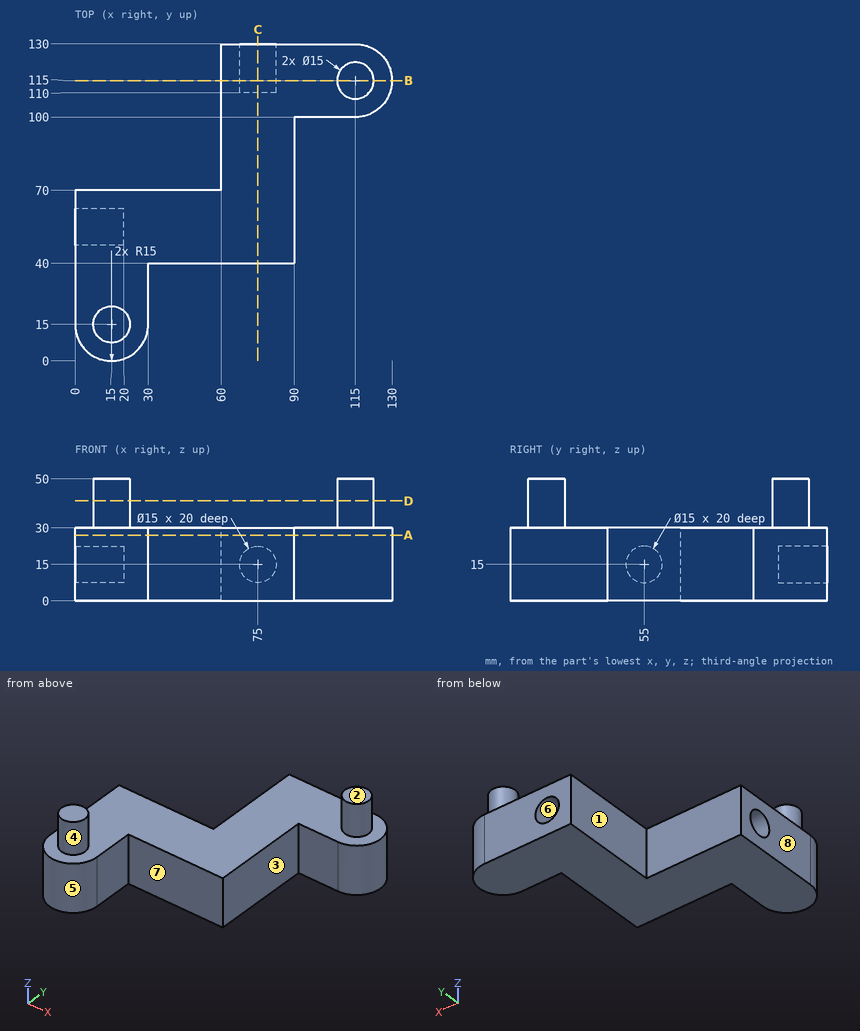
Drawing for the job (mm, zero at the part's lowest x, y, z). A direction names the side the tool comes from. Coordinates: 2 decimals unless noted, no trailing zeros. Write each loop counter-clockwise with the first axis right and the second up, starting at its lowest first coordinate (ties: lowest second). Pieces come first, ordered by that corner, then holes. Notation, with made-up numbers: (73.25, 76) -> (94.25, 76) arc R20 ccw to (94.25, 109) -> close; hole circle Ø11 at (8, 17.25). An arc over 180 degrees is marked (long way). One line per item, written item: value. Start each with the question number.
1) Flat gauge pins, fed straight in: pin 1 Ø15 at (y, z) = (63, 7.5) entering from +X; pin 2 Ø15 at (x, z) = (62.5, 17.5) entering from -Y; pin 3 Ø12.5 at (y, z) = (28.5, 8.5) entering from +X. Where does each tip first touch, or does it go through?
2) Which spindle directions (+Z, -Z, +X, -X, +Y, -Y) get a long thin tool onto all of the face, cutting with end or side? Do the marked faces 1, 2, 3, 4 and 5. Say none if no direction does.
3) Slice it at A-A on z = 27. Write the cut outline in (x, y).
4) Slice it at C-C on x = 75. Write the cut outline in (y, z), then the cut area to 3 significant figures.
5) Probe probe 1 along Z at (x, y) = (7, 55); probe 2 along X at (y, z) = (116, 15); probe 3 along Y at (x, z) = (38, 27.5). List the from-to ranges inside material, lowest first.
6) Slice it at B-B on y = 115. Write the cut outline in (x, z), then the cut area to 3 significant figures.
7) Slice it at D-D on z = 41. Write the cut outline in (x, y).
8) Pull direction X, two halves, no side cores. Call the marked faces 6, 7 and 8: +X half, -X half, draft (parallel to the pull), parting line (faces both ways), or undercut.
Answers follow:
1. pin 1: x = 90
1. pin 2: y = 40
1. pin 3: x = 30
2. face 1: +Z, -Z, -X, +Y
2. face 2: +Z, +X, -X, +Y, -Y
2. face 3: +Z, -Z, +X, -Y
2. face 4: +Z
2. face 5: +Z, -Z, -Y
3. outline: (0, 15) arc R15 ccw to (30, 15) -> (30, 40) -> (90, 40) -> (90, 100) -> (115, 100) arc R15 ccw to (115, 130) -> (60, 130) -> (60, 70) -> (0, 70) -> close
4. outline: (40, 0) -> (130, 0) -> (130, 7.5) -> (110, 7.5) -> (110, 22.5) -> (130, 22.5) -> (130, 30) -> (40, 30) -> close
4. area: 2,400 mm2
5. probe 1: 0 to 7.5, 22.5 to 30
5. probe 2: 60 to 67.5, 82.5 to 129.97
5. probe 3: 40 to 70
6. outline: (60, 0) -> (130, 0) -> (130, 30) -> (122.5, 30) -> (122.5, 50) -> (107.5, 50) -> (107.5, 30) -> (60, 30) -> close; hole circle Ø15 at (75, 15)
6. area: 2,220 mm2
7. outline: circle Ø15 at (15, 15); circle Ø15 at (115, 115)
8. face 6: undercut
8. face 7: draft
8. face 8: -X half
